from build123d import *

# Parameters (mm, degrees)
F0_W     = 139.885172
F0_H     = 18.295985
F1_DEPTH = 25
F3_D     = 8
F5_D     = 8


with BuildPart() as f1:
    # F0 (on Top) → F1 (new body)
    with BuildSketch(Plane.XY):
        with Locations((0.641361, 9.147992)):
            Rectangle(F0_W, F0_H)
    extrude(amount=F1_DEPTH)

    # F3 (through all)
    with Locations(Plane.XY.offset(25)):
        with Locations((-61.372835, 9.147992), (-46.562072, 9.147992), (-31.341393, 9.147992), (-16.530629, 9.147992), (0, 9.147992), (13.117687, 9.147992), (27.901655, 9.147992), (42.819589, 9.147992), (60.49981, 9.147992)):
            Hole(F3_D / 2)

    # F5 (through all)
    with Locations(Plane(origin=(0, 18.295985, 0), x_dir=(-1, 0, 0), z_dir=(0, 1, 0))):
        with Locations((-52.215707, 0), (53.392045, 0)):
            Hole(F5_D / 2)


solid = f1.part
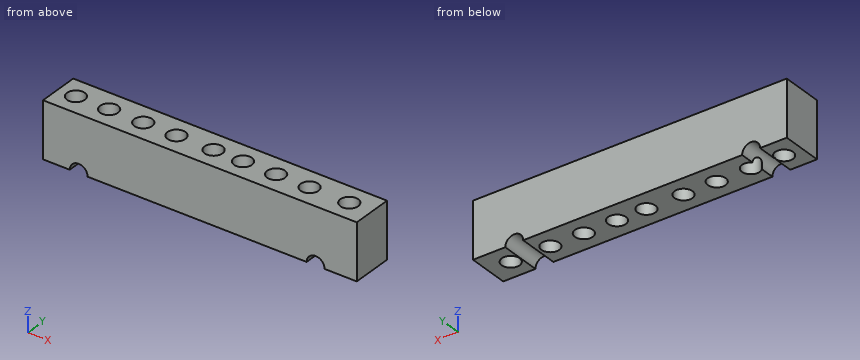
For this review, take the finished solid that the model builds, in its own axes (mm). Round coordinates to 2 decimals unless told otherwise and drop trailing zeros. Write each loop counter-clockwise with the first axis right and the second up, starting at its lowest first coordinate (ties: lowest second). Pieces come first, ordered by that corner, then holes. Notation, with made-up numbers: (-37.75, 17) - (-22.75, 17) arc R21 ccw to (-22.75, 38) - close; hole circle Ø5 at (-22, 82). An arc over 180 degrees is marked (long way). Write item = value, one per line. Start each with the question number.
1. Wall thickness on L1, parallel to Y at x = 0, z = 19.5; L2, parallel to X at y = 4.25, z = 1.5; L3, parallel to Y at x = 40, z = 22.25: over which ranges is each line inside the solid? List them lowest first.
2. For pin 1 Ø4 at (x, y) = (-29.5, 8) entering from +Z, flat-tipped, find the tip position at first contact; note if it passes through.
3. Consider section B-B on z = 21.75. Give the number of separate pieces and of enclosed holes in the cut face, plus the area to 3 significant figures.
4. Consider section A-A on x = 0. State the section outline as (y, z) points, plus the area to 3 significant figures.
5. Consider section C-C on x = 29. State the section outline as (y, z) points.
Evaluation:
q1.L1 = 0 to 5.15, 13.15 to 18.3
q1.L2 = -69.3 to -57.1, -49.68 to 48.51, 55.92 to 70.58
q1.L3 = 0 to 6.31, 11.99 to 18.3
q2.pin_1 = 25
q3.separate_pieces = 1
q3.enclosed_holes = 9
q3.area = 2,110 mm2
q4.outline = (0, 0) - (5.15, 0) - (5.15, 25) - (0, 25) - close; (13.15, 0) - (18.3, 0) - (18.3, 25) - (13.15, 25) - close
q4.area = 257 mm2
q5.outline = (0, 0) - (5.3, 0) - (5.3, 25) - (0, 25) - close; (12.99, 0) - (18.3, 0) - (18.3, 25) - (12.99, 25) - close
